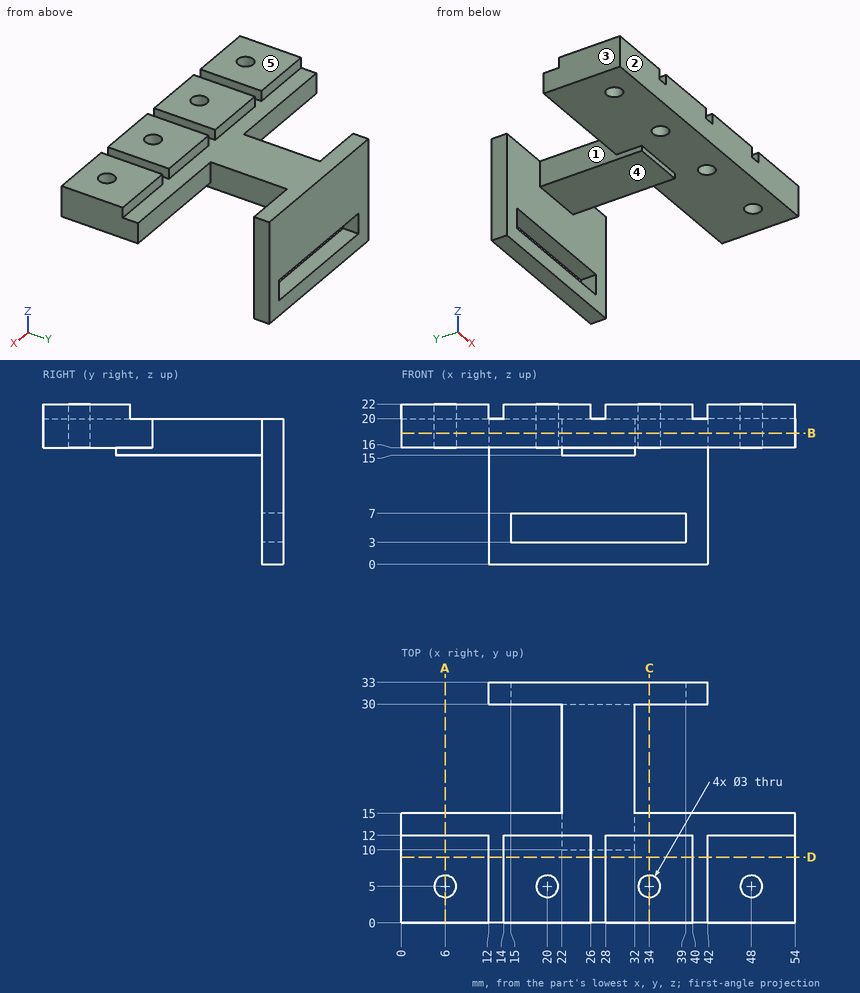
Drawing for the job (mm, zero at the part's lowest x, y, z). A direction names the side the tool comes from. Coordinates: 2 decimals unless noted, no trailing zeros. Loops run counter-clockwise (first coordinate to the right, second up) from the corner with the lowest first, then second, coordinate; pieces in that order, holes last. Notation, with made-up numbers: (33, 69) - (43, 69) arc R11 cw to (43, 73) - close; hole circle Ø1 at (13.25, 4.5). An arc over 180 degrees is marked (long way). Return JSON: item names as keys, results as strings.
1. Probe L1, parallel to Y at x = 34, z = 19.55; L2, parallel to Y at x = 6, z = 17.2; L3, parallel to X at y = 31.5, z = 3.5. List the from-to ranges inside material, lowest first. Write a range as from..to.
Result:
{"L1": "y = 0..3.5, 6.5..15, 30..33", "L2": "y = 0..3.5, 6.5..15", "L3": "x = 12..15, 39..42"}
2. Band-saw the part on A-A (x = 6). Give the cut face in (y, z), and give its area (3 significant figures).
Result:
{"outline": "(0, 16) - (3.5, 16) - (3.5, 22) - (0, 22) - close; (6.5, 16) - (15, 16) - (15, 20) - (12, 20) - (12, 22) - (6.5, 22) - close", "area": "66.0 mm2"}
3. Band-saw the part on D-D (y = 9). Give the cut face in (x, z), and give its area (3 significant figures).
Result:
{"outline": "(0, 16) - (54, 16) - (54, 22) - (42, 22) - (42, 20) - (40, 20) - (40, 22) - (28, 22) - (28, 20) - (26, 20) - (26, 22) - (14, 22) - (14, 20) - (12, 20) - (12, 22) - (0, 22) - close", "area": "312 mm2"}
4. Drop flat-ended pins along their axis: pin 1 (1.5 mm diameter, centred on y = 32, z = 4.5, fed in from +X); pin 2 (3 mm diameter, centred on x = 34.5, z = 14, fed in from -Y); pin 3 (1.5 mm diameter, centred on x = 31, y = 32, fed in from +Z); pin 4 (2.5 mm diameter, centred on x = 20, y = 5, fed in from -Z). Give the stop position or say it passes through.
Result:
{"pin 1": "stops at x = 42", "pin 2": "stops at y = 30", "pin 3": "stops at z = 20", "pin 4": "passes through"}
5. Band-saw the part on C-C (x = 34). Give the cut face in (y, z), and give its area (3 significant figures).
Result:
{"outline": "(0, 16) - (3.5, 16) - (3.5, 22) - (0, 22) - close; (6.5, 16) - (15, 16) - (15, 20) - (12, 20) - (12, 22) - (6.5, 22) - close; (30, 0) - (33, 0) - (33, 3) - (30, 3) - close; (30, 7) - (33, 7) - (33, 20) - (30, 20) - close", "area": "114 mm2"}
6. Band-saw the part on B-B (z = 18). Give the cut face in (x, y), and give its area (3 significant figures).
Result:
{"outline": "(0, 0) - (54, 0) - (54, 15) - (32, 15) - (32, 30) - (42, 30) - (42, 33) - (12, 33) - (12, 30) - (22, 30) - (22, 15) - (0, 15) - close; hole circle Ø3 at (6, 5); hole circle Ø3 at (20, 5); hole circle Ø3 at (34, 5); hole circle Ø3 at (48, 5)", "area": "1,020 mm2"}
7. Mould opens along Y. For the marked faces 1, 2 and 3 say: released by +Y, released by -Y, zero draft, split by the parting line, or undercut.
Result:
{"face 1": "undercut", "face 2": "released by -Y", "face 3": "zero draft"}
8. 3-axis set-ups, long thin cutter, end or side, ignore diameter. For the marked faces 4 and 5: which of +Z, -Z, +X, -X, +Y, -Y reach the whole face in a straight line?
Result:
{"face 4": "-Z, +X, -X, -Y", "face 5": "+Z, +X, -X, +Y, -Y"}
